from build123d import *

# Parameters (mm, degrees)
F0_R     = 7.5
F1_DEPTH = 38
F3_R     = 1.75
F4_R     = 8.25
F5_DEPTH = 1.5
F6_R     = 7.875
F7_DEPTH = 9


with BuildPart() as f1:
    # F0 (on Top) → F1 (new body)
    with BuildSketch(Plane.XY):
        Circle(F0_R)
    extrude(amount=F1_DEPTH)

    # F3
    f3_edges = [f1.edges().sort_by_distance(p)[0] for p in [
        (-7.5, 0, 38),
        (-7.5, 0, 0),
    ]]
    fillet(f3_edges, radius=F3_R)

    # F4 (on face) → F5 (join)
    with BuildSketch(Plane.XY.offset(38)):
        Circle(F4_R)
    extrude(amount=F5_DEPTH)

    # F6 (on face) → F7 (join)
    with BuildSketch(Plane.XY.offset(39.5)):
        Circle(F6_R)
    extrude(amount=F7_DEPTH)


solid = f1.part
Work out the finished part from the listing and answer in its coordinate system (mm). A direction names the side the tool comes from. Coordinates: 2 decimals unless noted, no trailing zeros. Loops run counter-clockwise (first coordinate to the right, second up) from the corner with the lowest first, then second, coordinate; pieces in that order, holes last. Notation, with made-up numbers: (-20, 35.25) -> (27, 35.25) arc R22 cw to (27, 48.25) -> close; hole circle Ø9 at (59.5, 36.25). An arc over 180 degrees is marked (long way). Write each question's results on one line, items separated by ' | '. Start each with the question number.
1) Find section A-A on y = 0. Determine the outline of the cut face in (x, z) (3 decimals), then the cut area to 3 significant figures.
2) The mould has two halves that part along Z. Classify faces 1 (the flat face through (3.6, -5.4, 38)), 2 (the flat face through (4, -7, 39.5)), 3 (the cylindrical face through (7.62, -3.16, 38.74)), 4 (the flat face through (0, 0, 0)): pulls with the +Z half, pulls with the -Z half, needs draft (parallel to the pull), parting line crosses it, or undercut.
3) Consider line 1 along Z through (x, y) = (-5.5, -5.5); line 2 along Z through (x, y) = (7, -0.5); line 3 along Z through (x, y) = (1, 6.5). Determine where each line is inside the solid, lowest interval first.
4) Flat-ended cylindrical pins translate along their axes: P1, Ø2, axis at y = 1, z = 26.5, coming from the -X side; P2, Ø4, axis at x = 2, z = 17.5, coming from the -Y side; P3, Ø1.5, axis at y = -6.5, z = 24.5, coming from the -X side. Find the tip coordinate at first contact, or state that the pin passes through.
5) For faces 5 (the flat face through (0, 0, 48.5)), 6 (the cylindrical face through (-1.025, 7.808, 43.937)), 7 (the cylindrical face through (-7.493, 0.33, 18.758)), determine the directions among +Z, -Z, +X, -X, +Y, -Y from which every point of the face is accessible in a straight line to the end or side of a thin tool.
Response values:
1) outline: (-8.25, 38) -> (-5.75, 38) arc R1.75 ccw to (-7.5, 36.25) -> (-7.5, 1.75) arc R1.75 ccw to (-5.75, 0) -> (5.75, 0) arc R1.75 ccw to (7.5, 1.75) -> (7.5, 36.25) arc R1.75 ccw to (5.75, 38) -> (8.25, 38) -> (8.25, 39.5) -> (7.875, 39.5) -> (7.875, 48.5) -> (-7.875, 48.5) -> (-7.875, 39.5) -> (-8.25, 39.5) -> close | area: 734 mm^2
2) face 1: undercut | face 2: pulls with the +Z half | face 3: needs draft | face 4: pulls with the -Z half
3) line 1: z = 38 to 48.5 | line 2: z = 0.54 to 37.46, 38 to 48.5 | line 3: z = 0.21 to 37.79, 38 to 48.5
4) P1: stops at x = -7.5 | P2: stops at y = -7.5 | P3: stops at x = -4.82
5) face 5: +Z, +X, -X, +Y, -Y | face 6: +Z | face 7: -Z
